The model under review builds one solid part; all positions refer to its coordinate system, in mm. Face numbers are marked on the shaded views. A direction names the side the tool comes from. Give positions to 0.01 mm unless a question says otherwise; leave off trailing zeros. Order: outer loops, then holes, each group sorted by start corner. A loop starts at its lowest first (then second) coordinate and runs counter-clockwise, first axis right, second up. Notation, with made-up numbers: (36.25, 26) - (66.25, 26) arc R11 ccw to (66.25, 38) - close; hole circle Ø8 at (71, 12.5). An arc over 180 degrees is marked (long way). Use CSV: the item, a comma, the result in double quotes.
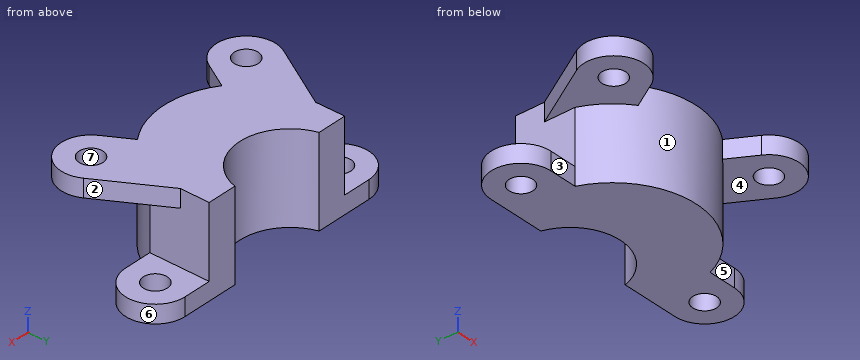
```python
from build123d import *

# Parameters (mm, degrees)
ESBO_O1_R                = 2
RESSALTO_EXTRUS_O1_DEPTH = 3
RESSALTO_EXTRUS_O2_DEPTH = 12
ESBO_O3_R                = 2
RESSALTO_EXTRUS_O3_DEPTH = 3


with BuildPart() as part:
    # Esboço1 → Ressalto-extrusão1 (new body)
    with BuildSketch(Plane.XY):
        with BuildLine():
            Line((-17.75, 4.940964043), (-13.099117311, 4.940964043))
            Line((-13.099117311, 4.940964043), (-8.154782397, 4.940964043))
            ThreePointArc((-8.154782397, 4.940964043), (0, -1.302389684), (8.154782397, 4.940964043))
            Line((8.154782397, 4.940964043), (13.099117311, 4.940964043))
            Line((13.099117311, 4.940964043), (17.75, 4.940964043))
            ThreePointArc((17.75, 4.940964043), (22.75, -0.059035957), (17.75, -5.059035957))
            Line((17.75, -5.059035957), (13.053970859, -5.059035957))
            ThreePointArc((13.053970859, -5.059035957), (0, -14), (-13.053970859, -5.059035957))
            Line((-13.053970859, -5.059035957), (-17.75, -5.059035957))
            ThreePointArc((-17.75, -5.059035957), (-22.75, -0.059035957), (-17.75, 4.940964043))
        make_face()
        with Locations((-17.75, -0.059035957)):
            Circle(ESBO_O1_R, mode=Mode.SUBTRACT)
        with Locations((17.75, -0.059035957)):
            Circle(ESBO_O1_R, mode=Mode.SUBTRACT)
    extrude(amount=RESSALTO_EXTRUS_O1_DEPTH)

    # Esboço2 → Ressalto-extrusão2 (add)
    with BuildSketch(Plane.XY.offset(3)):
        with BuildLine():
            Line((13.099117311, 4.940964043), (13.053970859, -5.059035957))
            ThreePointArc((13.053970859, -5.059035957), (0, -14), (-13.053970859, -5.059035957))
            Line((-13.053970859, -5.059035957), (-13.099117311, 4.940964043))
            Line((-13.099117311, 4.940964043), (-8.154782397, 4.940964043))
            ThreePointArc((-8.154782397, 4.940964043), (0, -1.302389684), (8.154782397, 4.940964043))
            Line((8.154782397, 4.940964043), (13.099117311, 4.940964043))
        make_face()
    extrude(amount=RESSALTO_EXTRUS_O2_DEPTH)

    # Esboço3 → Ressalto-extrusão3 (add)
    with BuildSketch(Plane.XY.offset(15)):
        with BuildLine():
            Line((13.077187708, 0.083527365), (8.154782397, -11.379785765))
            Line((8.154782397, -11.379785765), (10.671688275, -15.731898104))
            ThreePointArc((10.671688275, -15.731898104), (17.503141549, -17.55706828), (19.328311725, -10.725615007))
            Line((19.328311725, -10.725615007), (13.077187708, 0.083527365))
        make_face()
        with Locations((15, -13.228756555)):
            Circle(ESBO_O3_R, mode=Mode.SUBTRACT)
        with BuildLine():
            Line((-10.671688275, -15.731898104), (-8.154782397, -11.379785765))
            Line((-8.154782397, -11.379785765), (-13.077187708, 0.083527365))
            Line((-13.077187708, 0.083527365), (-19.328311725, -10.725615007))
            ThreePointArc((-19.328311725, -10.725615007), (-17.503141549, -17.55706828), (-10.671688275, -15.731898104))
        make_face()
        with Locations((-15, -13.228756555)):
            Circle(ESBO_O3_R, mode=Mode.SUBTRACT)
    extrude(amount=-RESSALTO_EXTRUS_O3_DEPTH)


solid = part.part
```
Item 1: Take a section at D-D, the plane x = 18.5. Give the boundary of the cut face in (y, z), and give its area (3 significant figures).
Results list:
outline,"(-16.8, 12) - (-9.29, 12) - (-9.29, 15) - (-16.8, 15) - close; (-5, 0) - (-1.91, 0) - (-1.91, 3) - (-5, 3) - close; (1.8, 0) - (4.88, 0) - (4.88, 3) - (1.8, 3) - close"
area,"41.1 mm2"
Item 2: Wall thickness on L1, parallel to Y at x = 17.75, z = 1.2; L2, parallel to X at y = -12, z = 13.25; L3, parallel to Z at x = -11.5, y = -8.5: over which ranges is each line inside the solid? List them lowest first.
Results list:
L1,"y = -5.06 to -2.06, 1.94 to 4.94"
L2,"x = -19.85 to -16.58, -13.42 to -8.51, -7.21 to 7.21, 8.51 to 13.42, 16.58 to 19.85"
L3,"z = 12 to 15"
Item 3: Mouldability with a two-part tool opening along Y and no side actions: class the marked faces 4, 5, 6 and 7 as pulls with the +Y half, pulls with the -Y half, needs draft (parallel to the pull), parting line crosses it, or undercut.
Results list:
face 4,"needs draft"
face 5,"pulls with the -Y half"
face 6,"parting line crosses it"
face 7,"undercut"
Item 4: Take a section at B-B, the plane y = -12.75. Give the boundary of the cut face in (x, z).
Results list:
outline,"(-19.98, 12) - (-16.94, 12) - (-16.94, 15) - (-19.98, 15) - close; (-13.06, 12) - (-8.95, 12) - (-8.95, 15) - (-13.06, 15) - close; (-5.78, 0) - (5.78, 0) - (5.78, 15) - (-5.78, 15) - close; (8.95, 12) - (13.06, 12) - (13.06, 15) - (8.95, 15) - close; (16.94, 12) - (19.98, 12) - (19.98, 15) - (16.94, 15) - close"
Item 5: Clearance check with flat-ended pins moving along their axes: pin 1 (8 mm diameter, centred on x = 19, y = 0, fed in from +Z); pin 2 (4 mm diameter, centred on y = -1, z = 8.5, fed in from +X); pin 3 (0.9 mm diameter, centred on x = -14.5, z = 2, fed in from -Y). State where each tip first meets the part, or that it passes through.
Results list:
pin 1,"stops at z = 3"
pin 2,"stops at x = 13.08"
pin 3,"stops at y = -5.06"
Item 6: Tool access review of the marked faces 1, 2 and 3: name each direction out of +Z, -Z, +X, -X, +Y, -Y from which nothing blocks a thin tool from reaching the whole face with its end or side.
Results list:
face 1,"-Z, -Y"
face 2,"+Z, +X, +Y"
face 3,"-Z, -X, -Y"
Item 7: Take a section at C-C, the plane z = 2.5. Give the boundary of the cut face in (x, y).
Results list:
outline,"(-17.75, -5.06) - (-13.05, -5.06) arc R14 ccw to (13.05, -5.06) - (17.75, -5.06) arc R5 ccw to (17.75, 4.94) - (8.15, 4.94) arc R8.45 cw to (-8.15, 4.94) - (-17.75, 4.94) arc R5 ccw to start; hole circle Ø4 at (-17.75, -0.06); hole circle Ø4 at (17.75, -0.06)"
Item 8: Take a section at A-A, the plane x = -14. Give the boundary of the cut face in (y, z).
Results list:
outline,"(-18.13, 12) - (-14.96, 12) - (-14.96, 15) - (-18.13, 15) - close; (-11.5, 12) - (-1.51, 12) - (-1.51, 15) - (-11.5, 15) - close; (-5.06, 0) - (4.94, 0) - (4.94, 3) - (-5.06, 3) - close"
